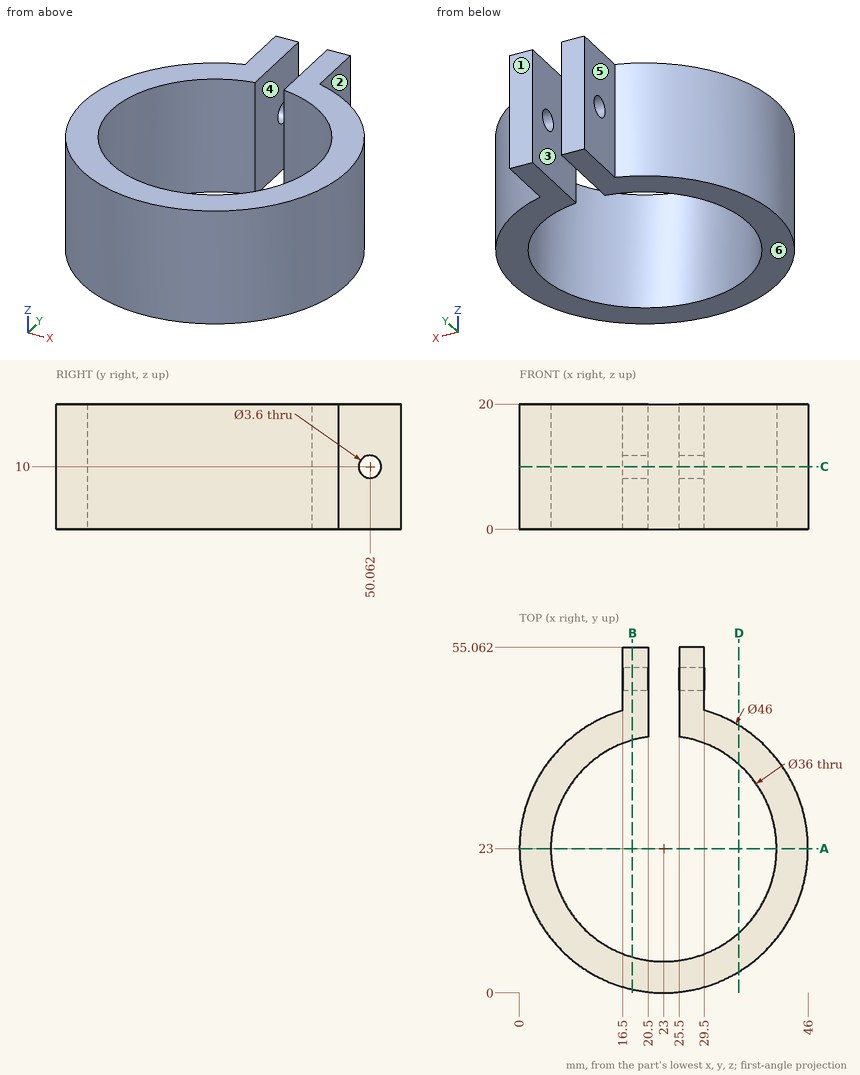
Here's the drawing with two shaded views (mm, measured from the low corner). I have some questions. A direction names the side the tool comes from. Coordinates: 2 decimals unless noted, no trailing zeros. Loops run counter-clockwise (first coordinate to the right, second up) from the corner with the lowest first, then second, coordinate; pieces in that order, holes last. Notation, with made-up numbers: (47, 54.5) -> (70, 54.5) arc R22 cw to (70, 86.5) -> close; hole circle Ø11 at (16.5, 35). An arc over 180 degrees is marked (long way). Put each result on its own line as item: value. Start each with the question number.
Q1. I'm going to push flat-ended pins straight in: P1, Ø3, axis at y = 52, z = 7, coming from the -X side; P2, Ø2, axis at y = 50.06, z = 10, coming from the +X side; P3, Ø6, axis at y = 50.06, z = 10, coming from the +X side; P4, Ø10, axis at x = 35, z = 14, coming from the +Y side. Where does each tip first touch, or does it pass through?
Q2. I want a section at C-C (z = 10). Write out the boundary of the cut face in (x, y) (1 decimal).
Q3. I want a section at B-B (x = 18). Write out the boundary of the cut face in (y, z).
Q4. If I drill on line 1 (X direction, y = 23, z = 11.5); line 2 (X direction, y = 52, z = 13); line 3 (Y direction, x = 23, z = 4.75), over which ranges is the centre line in solid material (lowest first)? Write a range as [from, to].
Q5. Thinking about a two-plate mould opening in X: for the marked faces 4, 5 and 6, which applies, pulls with the +X half, pulls with the -X half, needs draft (parallel to the pull), parting line crosses it, or undercut?
Q6. For the marked faces 1, 2 and 3, which set-ups out of +Z, -Z, +X, -X, +Y, -Y let a thin tool reach every point of the face, with its end or its side?
Q7. I want a section at D-D (x = 35). Write out the boundary of the cut face in (y, z), plus the area to 3 significant figures.
Q8. I want a section at A-A (y = 23). Write out the boundary of the cut face in (x, z).
Taken from the geometry:
1. P1: stops at x = 16.5
1. P2: passes through
1. P3: stops at x = 29.5
1. P4: stops at y = 44.91
2. outline: (16.5, 45.1) arc R23 ccw (long way) to (29.5, 45.1) -> (29.5, 48.3) -> (25.5, 48.3) -> (25.5, 40.8) arc R18 cw (long way) to (20.5, 40.8) -> (20.5, 48.3) -> (16.5, 48.3) -> close; (16.5, 51.9) -> (20.5, 51.9) -> (20.5, 55.1) -> (16.5, 55.1) -> close; (25.5, 51.9) -> (29.5, 51.9) -> (29.5, 55.1) -> (25.5, 55.1) -> close
3. outline: (0.55, 0) -> (5.71, 0) -> (5.71, 20) -> (0.55, 20) -> close; (40.29, 0) -> (55.06, 0) -> (55.06, 20) -> (40.29, 20) -> close; hole circle Ø3.6 at (50.06, 10)
4. line 1: x = [0, 5], [41, 46]
4. line 2: x = [16.5, 20.5], [25.5, 29.5]
4. line 3: y = [0, 5]
5. face 4: undercut
5. face 5: pulls with the -X half
5. face 6: needs draft
6. face 1: +Z, -Z, +X, -X, +Y
6. face 2: +Z, -Z, +X, +Y
6. face 3: +Z, -Z, +Y
7. outline: (3.38, 0) -> (9.58, 0) -> (9.58, 20) -> (3.38, 20) -> close; (36.42, 0) -> (42.62, 0) -> (42.62, 20) -> (36.42, 20) -> close
7. area: 248 mm2
8. outline: (0, 0) -> (5, 0) -> (5, 20) -> (0, 20) -> close; (41, 0) -> (46, 0) -> (46, 20) -> (41, 20) -> close
